Geometry: final body of the model. Coordinates: model frame, mm. Give positions to 0.01 mm unless a question says otherwise; leave off trailing zeros. Write each loop counter-clockwise with the first axis right and the second up, starting at its lowest first coordinate (ties: lowest second). Pieces come first, ordered by that corner, then holes. Notation, with made-up numbers: (-28.75, 65.25) - (25.25, 65.25) arc R32 ccw to (25.25, 97.25) - close; hole circle Ø6 at (2, -13.5). An arc over 180 degrees is marked (long way). One line per question, with ' | ' between items. Start each with the question number.
```python
from build123d import *

# Parameters (mm, degrees)
SKETCH1_R           = 12.75
SKETCH1_W           = 39.723964685
SKETCH1_H           = 62.830636574
SKETCH1_W_2         = 40.473473452
SKETCH1_H_2         = 59.45784712
SKETCH1_W_3         = 12.699510432
SKETCH1_H_3         = 12.334572549
SKETCH1_W_4         = 15.426505011
SKETCH1_H_4         = 13.414238347
BOSS_EXTRUDE1_DEPTH = 2


with BuildPart() as part:
    # Sketch1 → Boss-Extrude1 (new body)
    with BuildSketch(Plane.XY):
        with BuildLine():
            Line((61.855, -42.715), (-61.855, -42.715))
            ThreePointArc((-61.855, -42.715), (-63.269213562, -42.129213562), (-63.855, -40.715))
            Line((-63.855, -40.715), (-63.855, 40.715))
            ThreePointArc((-63.855, 40.715), (-63.269213562, 42.129213562), (-61.855, 42.715))
            Line((-61.855, 42.715), (61.855, 42.715))
            ThreePointArc((61.855, 42.715), (63.269213562, 42.129213562), (63.855, 40.715))
            Line((63.855, 40.715), (63.855, -40.715))
            ThreePointArc((63.855, -40.715), (63.269213562, -42.129213562), (61.855, -42.715))
        make_face()
        Circle(SKETCH1_R, mode=Mode.SUBTRACT)
        with Locations((-37.266991881, 0)):
            Rectangle(SKETCH1_W, SKETCH1_H, mode=Mode.SUBTRACT)
        with Locations((39.932411186, 0)):
            Rectangle(SKETCH1_W_2, SKETCH1_H_2, mode=Mode.SUBTRACT)
        with Locations((0, 23.561637286)):
            Rectangle(SKETCH1_W_3, SKETCH1_H_3, mode=Mode.SUBTRACT)
        with Locations((1.36349729, -26.254195002)):
            Rectangle(SKETCH1_W_4, SKETCH1_H_4, mode=Mode.SUBTRACT)
    extrude(amount=BOSS_EXTRUDE1_DEPTH)


solid = part.part
```
1) Line query: L1, parallel to X at y = -13, z = 0.4 (3 decimals); L2, parallel to Y at x = 0, z = 1.6 (3 decimals); L3, parallel to X at y = 26, z = 1.25 (3 decimals). Output: solid intervals per line, ascending.
2) Section A-A, the plane y = 6. Output: boundary loops of the cut face in (x, z) (3 decimals), plus the area to 3 significant figures.
3) Section D-D, the plane x = 0. Output: boundary loops of the cut face in (y, z) (3 decimals), plus the area to 3 significant figures.
4) Section B-B, the plane z = 0.4. Output: boundary loops of the cut face in (x, y) (3 decimals).
5) Section C-C, the plane x = -34.5. Output: boundary loops of the cut face in (y, z) (3 decimals).
6) Pull-direction query (Y, two-part tool) for faces 1 (the flat face through (15, 1, 0)), 2 (the cylindrical face through (-2.764, -12.447, 0.986)); classes: +Y half, -Y half, draft (parallel to the pull), parting line (faces both ways), or undercut.
Answer key:
1) L1: -63.855 to -57.129, -17.405 to 19.696, 60.169 to 63.855 | L2: -42.715 to -32.961, -19.547 to -12.75, 12.75 to 17.394, 29.729 to 42.715 | L3: -63.855 to -57.129, -17.405 to -6.35, 6.35 to 19.696, 60.169 to 63.855
2) outline: (-63.855, 0) - (-57.129, 0) - (-57.129, 2) - (-63.855, 2) - close; (-17.405, 0) - (-11.25, 0) - (-11.25, 2) - (-17.405, 2) - close; (11.25, 0) - (19.696, 0) - (19.696, 2) - (11.25, 2) - close; (60.169, 0) - (63.855, 0) - (63.855, 2) - (60.169, 2) - close | area: 50.0 mm^2
3) outline: (-42.715, 0) - (-32.961, 0) - (-32.961, 2) - (-42.715, 2) - close; (-19.547, 0) - (-12.75, 0) - (-12.75, 2) - (-19.547, 2) - close; (12.75, 0) - (17.394, 0) - (17.394, 2) - (12.75, 2) - close; (29.729, 0) - (42.715, 0) - (42.715, 2) - (29.729, 2) - close | area: 68.4 mm^2
4) outline: (-63.855, -40.715) arc R2 ccw to (-61.855, -42.715) - (61.855, -42.715) arc R2 ccw to (63.855, -40.715) - (63.855, 40.715) arc R2 ccw to (61.855, 42.715) - (-61.855, 42.715) arc R2 ccw to (-63.855, 40.715) - close; hole (-57.129, -31.415) - (-17.405, -31.415) - (-17.405, 31.415) - (-57.129, 31.415) - close; hole circle Ø25.5 at (0, 0); hole (-6.35, -32.961) - (9.077, -32.961) - (9.077, -19.547) - (-6.35, -19.547) - close; hole (-6.35, 17.394) - (6.35, 17.394) - (6.35, 29.729) - (-6.35, 29.729) - close; hole (19.696, -29.729) - (60.169, -29.729) - (60.169, 29.729) - (19.696, 29.729) - close
5) outline: (-42.715, 0) - (-31.415, 0) - (-31.415, 2) - (-42.715, 2) - close; (31.415, 0) - (42.715, 0) - (42.715, 2) - (31.415, 2) - close
6) face 1: draft | face 2: undercut
